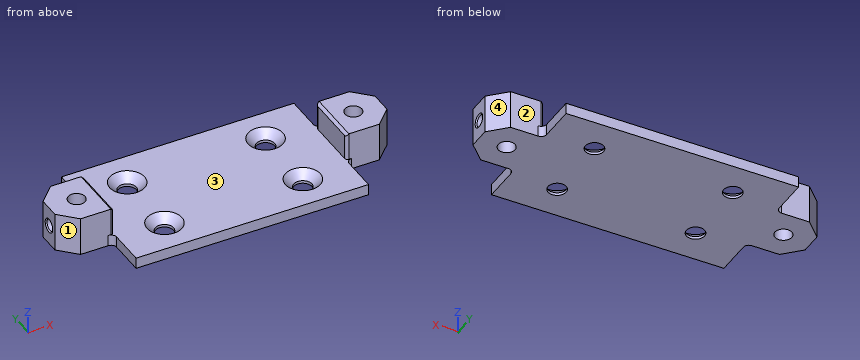
```python
from build123d import *

# Parameters (mm, degrees)
BOSS_EXTRUDE1_DEPTH                          = 4
CSK_FOR_M6_COUNTERSUNK_FLAT_HEAD_SCR_2_COUNT = 2
CSK_FOR_M6_COUNTERSUNK_FLAT_HEAD_SCR_2_PITCH = 25
CSK_FOR_M6_COUNTERSUNK_FLAT_HEAD_SCR_3_COUNT = 2
CSK_FOR_M6_COUNTERSUNK_FLAT_HEAD_SCR_3_PITCH = 55.901699437
CSK_FOR_M6_COUNTERSUNK_FLAT_HEAD_SCR_4_COUNT = 2
CSK_FOR_M6_COUNTERSUNK_FLAT_HEAD_SCR_4_PITCH = 50
SKETCH11_W                                   = 18
SKETCH11_H                                   = 20
BOSS_EXTRUDE4_DEPTH                          = 10
CHAMFER1_SIZE                                = 6
CUT_EXTRUDE5_REACH                           = 68.491
SKETCH12_R                                   = 3.05
FILLET2_R                                    = 2
CHAMFER2_SIZE                                = 1
FILLET3_R                                    = 1


# Read off the part's stored shape, not the designer's step: M5 Tapped Hole1
with BuildPart() as part:
    # Sketch1 → Boss-Extrude1 (new body)
    with BuildSketch(Plane.XY):
        Polygon((42, -25), (-42, -25), (-42, -10), (-60, -10), (-60, 10), (-42, 10), (-42, 25), (42, 25), (42, 10), (60, 10), (60, -10), (42, -10), align=None)
    extrude(amount=BOSS_EXTRUDE1_DEPTH)

    # Sketch10 → CSK for M6 Countersunk Flat Head Screw3 (revolve, cut)
    with BuildSketch(Plane(origin=(25, 12.5, 4), x_dir=(0, -1, 0), z_dir=(1, 0, 0))):
        Polygon((0, 0), (0, 4), (3.3, 4), (3.3, 3), (6.3, 0), align=None)
    csk_for_m6_countersunk_flat_head_screw3 = revolve(axis=Axis((25, 12.5, 10.35), (0, 0, -1)), mode=Mode.SUBTRACT)

    # CSK for M6 Countersunk Flat Head Scr 2: CSK for M6 Countersunk Flat Head Screw3 ×2
    with Locations(*[(0, -i * CSK_FOR_M6_COUNTERSUNK_FLAT_HEAD_SCR_2_PITCH, 0) for i in range(1, CSK_FOR_M6_COUNTERSUNK_FLAT_HEAD_SCR_2_COUNT)]):
        add(csk_for_m6_countersunk_flat_head_screw3, mode=Mode.SUBTRACT)

    # CSK for M6 Countersunk Flat Head Scr 3: CSK for M6 Countersunk Flat Head Screw3 ×2
    with Locations(*[Vector(-0.894427190999916, -0.447213595499958, 0) * (i * CSK_FOR_M6_COUNTERSUNK_FLAT_HEAD_SCR_3_PITCH) for i in range(1, CSK_FOR_M6_COUNTERSUNK_FLAT_HEAD_SCR_3_COUNT)]):
        add(csk_for_m6_countersunk_flat_head_screw3, mode=Mode.SUBTRACT)

    # CSK for M6 Countersunk Flat Head Scr 4: CSK for M6 Countersunk Flat Head Screw3 ×2
    with Locations(*[(-i * CSK_FOR_M6_COUNTERSUNK_FLAT_HEAD_SCR_4_PITCH, 0, 0) for i in range(1, CSK_FOR_M6_COUNTERSUNK_FLAT_HEAD_SCR_4_COUNT)]):
        add(csk_for_m6_countersunk_flat_head_screw3, mode=Mode.SUBTRACT)

    # Sketch11 → Boss-Extrude4 (add)
    with BuildSketch(Plane.XY.offset(4)):
        with Locations((51, 0)):
            Rectangle(SKETCH11_W, SKETCH11_H)
        with Locations((-51, 0)):
            Rectangle(SKETCH11_W, SKETCH11_H)
    extrude(amount=BOSS_EXTRUDE4_DEPTH)

    # Chamfer1
    chamfer1_edges = [part.edges().sort_by_distance(p)[0] for p in [
        (60, 10, 7),
        (60, -10, 7),
        (-60, -10, 7),
        (-60, 10, 7),
    ]]
    chamfer(chamfer1_edges, length=CHAMFER1_SIZE)

    # Sketch12 → Cut-Extrude5 (cut, up to next)
    with BuildSketch(Plane.XY.offset(14), mode=Mode.PRIVATE) as cut_extrude5_sk1:
        with Locations((50, 0)):
            Circle(SKETCH12_R)
    cut_extrude5_tool1 = extrude(cut_extrude5_sk1.sketch, amount=-CUT_EXTRUDE5_REACH, mode=Mode.PRIVATE) & part.part
    # Sketch12 → Cut-Extrude5 (cut, up to next)
    with BuildSketch(Plane.XY.offset(14), mode=Mode.PRIVATE) as cut_extrude5_sk2:
        with Locations((-50, 0)):
            Circle(SKETCH12_R)
    cut_extrude5_tool2 = extrude(cut_extrude5_sk2.sketch, amount=-CUT_EXTRUDE5_REACH, mode=Mode.PRIVATE) & part.part
    add(cut_extrude5_tool1.solids().sort_by_distance((50, 0, 14))[0], mode=Mode.SUBTRACT)
    add(cut_extrude5_tool2.solids().sort_by_distance((-50, 0, 14))[0], mode=Mode.SUBTRACT)

    # Fillet2
    fillet2_edges = [part.edges().sort_by_distance(p)[0] for p in [
        (42, 10, 2),
        (42, -10, 2),
        (-42, -10, 2),
        (-42, 10, 2),
    ]]
    fillet(fillet2_edges, radius=FILLET2_R)

    # Chamfer2
    chamfer2_edges = [part.edges().sort_by_distance(p)[0] for p in [
        (42, 0, 14),
        (-42, 0, 14),
    ]]
    chamfer(chamfer2_edges, length=CHAMFER2_SIZE)

    # Fillet3
    fillet3_edges = [part.edges().sort_by_distance(p)[0] for p in [
        (42, 10, 8.5),
        (42, -10, 8.5),
        (-42, 10, 8.5),
        (-42, -10, 8.5),
    ]]
    fillet(fillet3_edges, radius=FILLET3_R)

    # M5 Tapped Hole1 outline → M5 Tapped Hole1 (revolve, cut)
    with BuildSketch(Plane.YX.offset(-7)):
        Polygon((2.1, -59.575), (2.1, -52.211448723), (0, -52.211448723), (0, -60), (2.525, -60), align=None)
        Polygon((0, 52.211448731), (2.1, 52.211448731), (2.1, 59.575), (2.525, 60), (0, 60), align=None)
    revolve(axis=Axis((0, 0, 7), (1, 0, 0)), mode=Mode.SUBTRACT)


solid = part.part
```
CAD build for the part. Positions are in the model's coordinates, mm. Face numbers are marked on the shaded views. Round coordinates to 2 decimals unless told otherwise and drop trailing zeros. Write each loop counter-clockwise with the first axis right and the second up, starting at its lowest first coordinate (ties: lowest second). Pieces come first, ordered by that corner, then holes. Notation, with made-up numbers: (-32, -32) - (2, -32) arc R14 ccw to (2, -20) - close; hole circle Ø8 at (-35.75, 58.5). An arc over 180 degrees is marked (long way). Write item = value, one per line. Start each with the question number.
Q1. Probe L1, parallel to X at y = -12.5, z = 0.5; L2, parallel to Y at x = -50, z = 7.25; L3, parallel to Z at x = 41.5, y = -8. List the from-to ranges inside material, lowest first. Write a range as from..to.
Q2. Band-saw the part on A-A (x = 50). Give the cut face in (y, z), then the cut area to 3 significant figures.
Q3. Drop flat-ended pins along their axis: pin 1 (3 mm diameter, centred on y = 20, z = 1.5, fed in from -X); pin 2 (2.5 mm diameter, centred on y = 0, z = 7, fed in from +X); pin 3 (10.5 mm diameter, centred on x = 25, y = -12.5, fed in from +Z). Give the stop position or say it passes through.
Q4. Mould opens along X. For the marked faces 1, 2, 3 and 4 say: pulls with the +X half, pulls with the -X half, needs draft (parallel to the pull), parting line crosses it, or undercut.
Q5. Band-saw the part on C-C (y = 0). Count the separate pieces of the cut face and the enclosed holes in it, then the cut area to 3 significant figures.
Q6. Band-saw the part on D-D (x = -39). Give the cut face in (y, z).
Q7. Band-saw the part on B-B (z = 7). Give the cut face in (x, y) (3 decimals).
Answers below:
q1.L1 = -42..-28.3, -21.7..21.7, 28.3..42
q1.L2 = -10..-3.05, 3.05..10
q1.L3 = 0..4
q2.outline = (-10, 0) - (-3.05, 0) - (-3.05, 14) - (-10, 14) - close; (3.05, 0) - (10, 0) - (10, 14) - (3.05, 14) - close
q2.area = 195 mm2
q3.pin_1 = -42
q3.pin_2 = 47.22
q3.pin_3 = 2.95
q4.face_1 = pulls with the -X half
q4.face_2 = needs draft
q4.face_3 = undercut
q4.face_4 = pulls with the +X half
q5.separate_pieces = 5
q5.enclosed_holes = 0
q5.area = 609 mm2
q6.outline = (-25, 0) - (25, 0) - (25, 4) - (-25, 4) - close
q7.outline = (-60, -4) - (-54, -10) - (-43, -10) arc R1 ccw to (-42, -9) - (-42, 9) arc R1 ccw to (-43, 10) - (-54, 10) - (-60, 4) - (-60, 2.525) - (-59.575, 2.1) - (-52.212, 2.1) arc R3.05 cw (long way) to (-52.212, -2.1) - (-59.575, -2.1) - (-60, -2.525) - close; (42, -9) arc R1 ccw to (43, -10) - (54, -10) - (60, -4) - (60, -2.525) - (59.575, -2.1) - (52.212, -2.1) arc R3.05 cw (long way) to (52.212, 2.1) - (59.575, 2.1) - (60, 2.525) - (60, 4) - (54, 10) - (43, 10) arc R1 ccw to (42, 9) - close
